from build123d import *

# Parameters (mm, degrees)
F0_W     = 300
F0_H     = 200
F0_R     = 60
F1_DEPTH = 30
F2_W     = 25
F2_H     = 200
F3_DEPTH = 10
F5_DEPTH = 200
F6_R     = 5
F7_DEPTH = 15


with BuildPart() as f1:
    # F0 (on Top) → F1 (new body)
    with BuildSketch(Plane.XY):
        Rectangle(F0_W, F0_H)
        Circle(F0_R, mode=Mode.SUBTRACT)
    extrude(amount=F1_DEPTH)

    # F2 (on face) → F3 (cut)
    with BuildSketch(Plane.XY.offset(30)):
        with Locations((-102.5, 0)):
            Rectangle(F2_W, F2_H)
        Rectangle(F2_W, F2_H)
        with BuildLine():
            Line((-12.5, -58.683473), (-12.5, -100))
            Line((-12.5, -100), (12.5, -100))
            Line((12.5, -100), (12.5, -58.683473))
            ThreePointArc((12.5, -58.683473), (0, -60), (-12.5, -58.683473))
        make_face()
        with BuildLine():
            Line((12.5, 100), (-12.5, 100))
            Line((-12.5, 100), (-12.5, 58.683473))
            ThreePointArc((-12.5, 58.683473), (0, 60), (12.5, 58.683473))
            Line((12.5, 58.683473), (12.5, 100))
        make_face()
    extrude(amount=-F3_DEPTH, mode=Mode.SUBTRACT)

    # F4 (on face) → F5 (cut, through all)
    with BuildSketch(Plane.XZ.offset(100)):
        Polygon((115, 30), (90, 30), (84.226497, 20), (120.773503, 20), align=None)
    extrude(amount=-F5_DEPTH, mode=Mode.SUBTRACT)

    # F6 (on face) → F7 (join)
    with BuildSketch(Plane.YZ.offset(150)):
        with Locations((0, 15)):
            Circle(F6_R)
    extrude(amount=F7_DEPTH)


solid = f1.part
Can you work these out from the model? Positions are in its coordinate system, mm. A direction names the side the tool comes from. Give positions to 0.01 mm unless a question says otherwise; leave off trailing zeros. Loops run counter-clockwise (first coordinate to the right, second up) from the corner with the lowest first, then second, coordinate; pieces in that order, holes last. Notation, with made-up numbers: M 38.5,-22.5 L 79.5,-22.5 A9 ccw 79.5,-11.5 Z; hole C 77,-23 d11. An arc over 180 degrees is marked long. One line per item, written item: value. Start each with the question number.
1) On a 3-axis mill with a long thin cutter (end or side, diameter ignored), from which of +Z, -Z, +X, -X, +Y, -Y can I reach the whole of each face in a straight line? I mean faces 1 (the face through (-133, 1, 30)), 2 (the face through (0, 80, 20)), 3 (the face through (157.4, -1.08, 10.12)). Say none if no direction works.
2) If we section it at D-D, the plane y = 74.5: Write out the boundary of the cut face in (x, z), and give its area (3 significant figures).
3) If we section it at A-A, the plane y = 0: Write out the boundary of the cut face in (x, z).
4) If we section it at B-B, the plane x = 0: Write out the boundary of the cut face in (y, z), and give its area (3 significant figures).
5) If I drill on line 1 (Y direction, x = 0, z = 19); line 2 (X direction, y = 0, z = 15.75); line 3 (X direction, y = -21, z = 28), over which ranges is the centre line in solid material (lowest first)? Write a range as [from, to].
6) Thinking about a two-plate mould opening in X: for faces 4 (the face through (-12.5, -79, 25)), 5 (the face through (-150, -1, 15)), 6 (the face through (-60.4, 1.4, 30)), which applies, +X half, -X half, draft (parallel to the pull), parting line (faces both ways), or undercut?
7) I'm going to push flat-ended pins straight in: pin 1 (3 mm diameter, centred on y = 51, z = 17, fed in from +X); pin 2 (7.5 mm diameter, centred on x = 3.5, y = 82.5, fed in from +Z). Where does each tip first touch, or does it pass through?
8) If we section it at C-C, the plane z = 15: Write out the boundary of the cut face in (x, y), and give its area (3 significant figures).
Completed:
1. face 1: +Z, +X, -X, +Y, -Y
1. face 2: +Z, +Y, -Y
1. face 3: +X
2. outline: M -150,0 L 150,0 L 150,30 L 115,30 L 120.77,20 L 84.23,20 L 90,30 L 12.5,30 L 12.5,20 L -12.5,20 L -12.5,30 L -90,30 L -90,20 L -115,20 L -115,30 L -150,30 Z
2. area: 8,190 mm^2
3. outline: M -150,0 L -60,0 L -60,30 L -90,30 L -90,20 L -115,20 L -115,30 L -150,30 Z; M 60,0 L 150,0 L 150,10 L 165,10 L 165,20 L 150,20 L 150,30 L 115,30 L 120.77,20 L 84.23,20 L 90,30 L 60,30 Z
4. outline: M -100,0 L -60,0 L -60,20 L -100,20 Z; M 60,0 L 100,0 L 100,20 L 60,20 Z
4. area: 1,600 mm^2
5. line 1: y = [-100, -60], [60, 100]
5. line 2: x = [-150, -60], [60, 165]
5. line 3: x = [-150, -115], [-90, -56.2], [56.2, 88.85], [116.15, 150]
6. face 4: undercut
6. face 5: -X half
6. face 6: draft
7. pin 1: stops at x = 150
7. pin 2: stops at z = 20
8. outline: M -150,-100 L 150,-100 L 150,-5 L 165,-5 L 165,5 L 150,5 L 150,100 L -150,100 Z; hole C 0,0 d120
8. area: 48,800 mm^2
